```python
from build123d import *

# Parameters (mm, degrees)
SKETCH3_R           = 266.7
BOSS_EXTRUDE1_DEPTH = 76.2
SKETCH4_R           = 241.3
SKETCH4_R_2         = 215.9
CUT_EXTRUDE1_DEPTH  = 25.4
SKETCH5_R           = 254
SKETCH5_R_2         = 203.2
CUT_EXTRUDE2_DEPTH  = 25.4
SKETCH6_W           = 43.18
SKETCH6_H           = 127
BOSS_EXTRUDE2_DEPTH = 101.6
BOSS_EXTRUDE3_START = -43.18
BOSS_EXTRUDE3_DEPTH = 43.18
BOSS_EXTRUDE4_DEPTH = 43.18
SKETCH7_R           = 38.1
CUT_EXTRUDE3_DEPTH  = 566.878709972


with BuildPart() as part:
    # Sketch3 → Boss-Extrude1 (new body)
    with BuildSketch(Plane(origin=(0, 0, 0), x_dir=(1, 0, 0), z_dir=(0, 1, 0))):
        with Locations(Location((0, 0, 0), (0, 0, 90))):
            Circle(SKETCH3_R)
    extrude(amount=BOSS_EXTRUDE1_DEPTH)

    # Sketch4 → Cut-Extrude1 (cut)
    with BuildSketch(Plane.XZ):
        with Locations(Location((0, 0, 0), (0, 0, 270))):
            Circle(SKETCH4_R)
        with Locations(Location((0, 0, 0), (0, 0, 270))):
            Circle(SKETCH4_R_2, mode=Mode.SUBTRACT)
    extrude(amount=-CUT_EXTRUDE1_DEPTH, mode=Mode.SUBTRACT)

    # Sketch5 → Cut-Extrude2 (cut)
    with BuildSketch(Plane.XZ.offset(-25.4)):
        with Locations(Location((0, 0, 0), (0, 0, 270))):
            Circle(SKETCH5_R)
        with Locations(Location((0, 0, 0), (0, 0, 270))):
            Circle(SKETCH5_R_2, mode=Mode.SUBTRACT)
    extrude(amount=-CUT_EXTRUDE2_DEPTH, mode=Mode.SUBTRACT)

    # Sketch6 → Boss-Extrude2 (add)
    with BuildSketch(Plane(origin=(0, 76.2, 0), x_dir=(1, 0, 0), z_dir=(0, 1, 0))):
        with Locations((148.59, 0)):
            Rectangle(SKETCH6_W, SKETCH6_H)
        with Locations((-148.59, 0)):
            Rectangle(SKETCH6_W, SKETCH6_H)
    extrude(amount=BOSS_EXTRUDE2_DEPTH)

    # Sketch8 → Boss-Extrude3 (add)
    with BuildSketch(Plane.ZY.offset(170.18).offset(BOSS_EXTRUDE3_START)):
        with BuildLine():
            Line((-63.5, 177.8), (63.5, 177.8))
            ThreePointArc((63.5, 177.8), (0, 241.3), (-63.5, 177.8))
        make_face()
    extrude(amount=BOSS_EXTRUDE3_DEPTH)

    # Sketch10 → Boss-Extrude4 (add)
    with BuildSketch(Plane(origin=(170.18, 0, 0), x_dir=(0, 0, -1), z_dir=(1, 0, 0))):
        with BuildLine():
            Line((63.5, 177.8), (-63.5, 177.8))
            ThreePointArc((-63.5, 177.8), (0, 241.3), (63.5, 177.8))
        make_face()
    extrude(amount=-BOSS_EXTRUDE4_DEPTH)

    # Sketch7 → Cut-Extrude3 (cut, through all)
    with BuildSketch(Plane(origin=(170.18, 0, 0), x_dir=(0, 0, -1), z_dir=(1, 0, 0))):
        with Locations((0, 177.8)):
            Circle(SKETCH7_R)
    extrude(amount=-CUT_EXTRUDE3_DEPTH, mode=Mode.SUBTRACT)


solid = part.part
```
The model under review builds one solid part; all positions refer to its coordinate system, in mm. A direction names the side the tool comes from. Round coordinates to 2 decimals unless told otherwise and drop trailing zeros. Write each loop counter-clockwise with the first axis right and the second up, starting at its lowest first coordinate (ties: lowest second). Pieces come first, ordered by that corner, then holes. Notation, with made-up numbers: (-28, 52.5) -> (6, 52.5) arc R9 cw to (6, 64.5) -> close; hole circle Ø11 at (86.25, 66.5). An arc over 180 degrees is marked (long way). Use CSV: the item, a comma, the result in double quotes.
Q1. For faces 4 (the flat face through (-127, 142, -15)), 5 (the flat face through (-149, 126, -63.5)), 6 (the flat face through (-127, 25.4, -159)), 7 (the flat face through (170.18, 142, -15)), 8 (the cylindrical face through (10.61, 12.522, 241.067)), list the 3-axis set-ups (+Z, -Z, +X, -X, +Y, -Y) from which the entire face can be reached by the end or side of a thin tool; tool diameter is ignored.
Checks:
face 4,"+Z, -Z, +Y"
face 5,"-Z, +X, -X, +Y"
face 6,"none"
face 7,"+Z, -Z, +X, +Y"
face 8,"-Y"
Q2. Consider section D-D (x = 0). Give the boundary of the cut face in (y, z), then the cut area to 3 significant figures.
Checks:
outline,"(0, -266.7) -> (76.2, -266.7) -> (76.2, 266.7) -> (0, 266.7) -> (0, 241.3) -> (25.4, 241.3) -> (25.4, 254) -> (50.8, 254) -> (50.8, 203.2) -> (25.4, 203.2) -> (25.4, 215.9) -> (0, 215.9) -> (0, -215.9) -> (25.4, -215.9) -> (25.4, -203.2) -> (50.8, -203.2) -> (50.8, -254) -> (25.4, -254) -> (25.4, -241.3) -> (0, -241.3) -> close"
area,"36,800 mm²"
Q3. Consider section B-B (x = 153). Give the boundary of the cut face in (y, z), then the cut area to 3 significant figures.
Checks:
outline,"(0, -218.45) -> (76.2, -218.45) -> (76.2, -63.5) -> (177.8, -63.5) arc R63.5 ccw to (177.8, 63.5) -> (76.2, 63.5) -> (76.2, 218.45) -> (0, 218.45) -> (0, 186.59) -> (25.4, 186.59) -> (25.4, 202.75) -> (50.8, 202.75) -> (50.8, 133.72) -> (25.4, 133.72) -> (25.4, 152.33) -> (0, 152.33) -> (0, -152.33) -> (25.4, -152.33) -> (25.4, -133.72) -> (50.8, -133.72) -> (50.8, -202.75) -> (25.4, -202.75) -> (25.4, -186.59) -> (0, -186.59) -> close; hole circle Ø76.2 at (177.8, 0)"
area,"42,700 mm²"
Q4. For pin 1 Ø8 at (y, z) = (184.5, -48.5) entering from +X; pin 2 Ø21.5 at (x, y) = (-158.5, 148) entering from +Z; pin 3 Ø1 at (x, y) = (202.5, 64.5) entering from -Z; pin 4 Ø1.5 at (x, y) = (-19.5, 77.5) entering from -Z, all flat-tipped, find the tip position at first contact; note any pin that passes through.
Checks:
pin 1,"x = 170.18"
pin 2,"z = 63.5"
pin 3,"z = -174.14"
pin 4,"through"
Q5. Mouldability with a two-part tool opening along Z and no side actions: class faces 1 (the flat face through (-170.18, 142, -15)), 2 (the cylindrical face through (148.892, 241.285, 1.396)), 3 (the cylindrical face through (145.915, 12.522, 159.127)) as released by +Z, released by -Z, zero draft, split by the parting line, or undercut.
Checks:
face 1,"zero draft"
face 2,"split by the parting line"
face 3,"undercut"
Q6. Consider section A-A (y = 91). Give the boundary of the cut face in (x, z).
Checks:
outline,"(-170.18, -63.5) -> (-127, -63.5) -> (-127, 63.5) -> (-170.18, 63.5) -> close; (127, -63.5) -> (170.18, -63.5) -> (170.18, 63.5) -> (127, 63.5) -> close"
Q7. To check wall thickness, follow probe 1 along X at (y, z) = (33, 0); probe 2 along X at (y, z) = (11, 0); probe 3 along X at (y, z) = (89, -12). State the ranges of each line that lie inside material, in increasing order. Write a range as [from, to].
Checks:
probe 1,"[-266.7, -254], [-203.2, 203.2], [254, 266.7]"
probe 2,"[-266.7, -241.3], [-215.9, 215.9], [241.3, 266.7]"
probe 3,"[-170.18, -127], [127, 170.18]"
Q8. Consider section C-C (y = 17). Give the boundary of the cut face in (x, z), then the cut area to 3 significant figures.
Checks:
outline,"circle Ø533.4 at (0, 0); circle Ø431.8 at (0, 0); hole circle Ø482.6 at (0, 0)"
area,"187,000 mm²"
